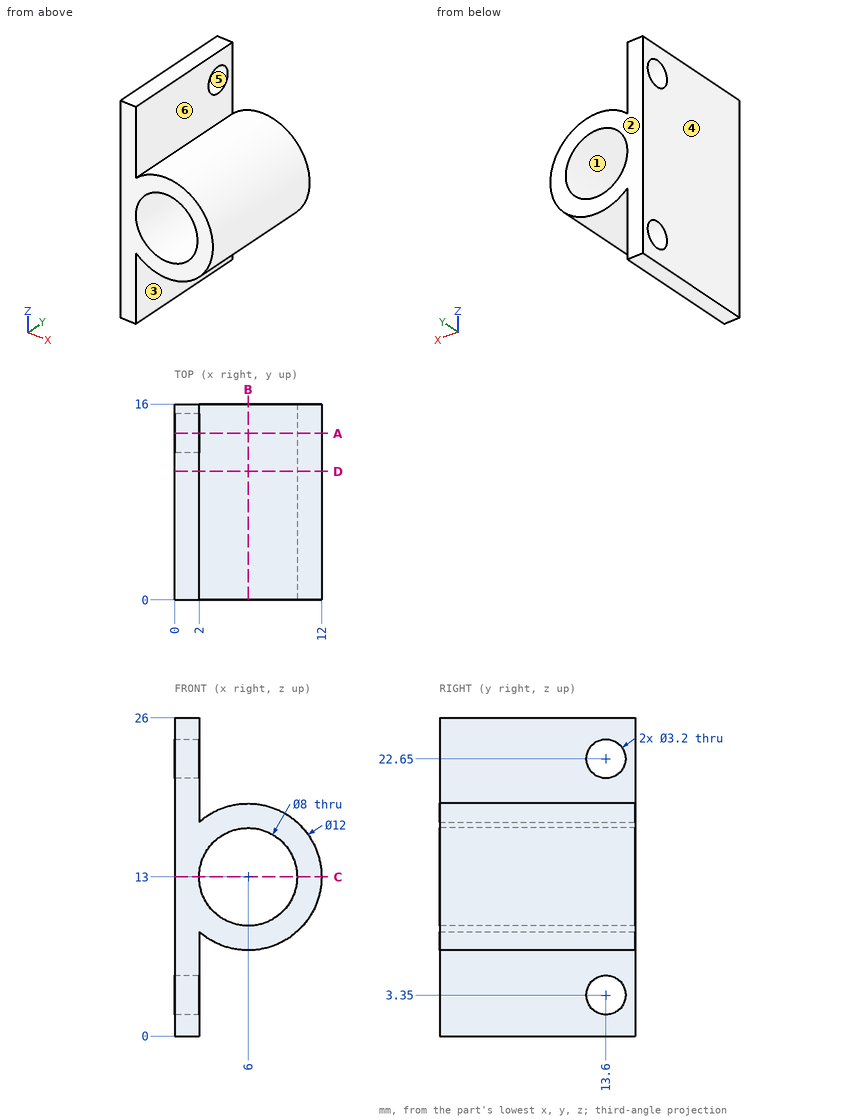
The drawing under review shows one solid part. Ordinate dimensions are in mm from its lowest x, y, z. A direction names the side the tool comes from. Coordinates: 2 decimals unless noted, no trailing zeros. Loops run counter-clockwise (first coordinate to the right, second up) from the corner with the lowest first, then second, coordinate; pieces in that order, holes last. Notation, with made-up numbers: M 47,-7 L 77,-7 A35 cw 77,31 Z; hole C 37,36.5 d6. An arc over 180 degrees is marked long. Use one line per item in the form item = value.
(1) For the marked faces 5 and 6, list the 3-axis set-ups (+Z, -Z, +X, -X, +Y, -Y) from which the entire face can be reached by the end or side of a thin tool; tool diameter is ignored.
Return value:
face_5 = +X, -X
face_6 = +Z, +Y, -Y
(2) For line 1 along Y through (x, z) = (1.55, 22.65); line 2 along Z through (x, y) = (1.25, 14.75); line 3 along X through (y, z) = (9.5, 5.75), list the stretches that pass through material, from the lowest coordinate up. Write a range as from..to.
Return value:
line_1 = 0..12, 15.2..16
line_2 = 0..2.24, 4.46..21.54, 23.76..26
line_3 = 0..2
(3) Draft analysis for pull direction X (two halves, no side actions). For the marked faces 1, 2, 3 and 4, state which applies: pulls with the +X half, pulls with the -X half, needs draft (parallel to the pull), parting line crosses it, or undercut.
Return value:
face_1 = undercut
face_2 = needs draft
face_3 = undercut
face_4 = pulls with the -X half
(4) Consider section D-D (y = 10.5). Write out the cut boundary in (x, z), and give its area (3 significant figures).
Return value:
outline = M 0,0 L 2,0 L 2,8.53 A6 ccw long 2,17.47 L 2,26 L 0,26 Z; hole C 6,13 d8
area = 102 mm2
(5) Consider section B-B (x = 6). Write out the cut boundary in (y, z).
Return value:
outline = M 0,7 L 16,7 L 16,9 L 0,9 Z; M 0,17 L 16,17 L 16,19 L 0,19 Z
(6) Consider section A-A (y = 13.6). Write out the cut boundary in (x, z).
Return value:
outline = M 0,0 L 2,0 L 2,1.75 L 0,1.75 Z; M 0,4.95 L 2,4.95 L 2,8.53 A6 ccw long 2,17.47 L 2,21.05 L 0,21.05 Z; M 0,24.25 L 2,24.25 L 2,26 L 0,26 Z; hole C 6,13 d8
(7) Consider section C-C (z = 13). Write out the cut boundary in (x, y).
Return value:
outline = M 0,0 L 2,0 L 2,16 L 0,16 Z; M 10,0 L 12,0 L 12,16 L 10,16 Z
(8) Clearance check with flat-ended pins moving along their axes: P1, Ø1, axis at x = 9.5, y = 10.5, coming from the -Z side; P2, Ø5, axis at y = 13.6, z = 3.35, coming from the +X side; P3, Ø9.5, axis at y = 5, z = 23, coming from the +X side (1 decimal); P4, Ø1.9, axis at y = 13.6, z = 22.65, coming from the +X side. State where each tip first meets the part, or that it passes through.
Return value:
P1 = 7.8
P2 = 2
P3 = 8.9
P4 = through
